The figure shows three views and two pictorial views of one solid part (mm, origin at its lowest corner). Answer the questions. A direction names the side the tool comes from. Coordinates: 2 decimals unless noted, no trailing zeros. Loops run counter-clockwise (first coordinate to the right, second up) from the corner with the lowest first, then second, coordinate; pieces in that order, holes last. Notation, with made-up numbers: M 79,16.25 L 94,16.25 A25 cw 94,51.25 Z; hole C 18,-11 d8. An arc over 180 degrees is marked long. Write each question's results on one line, items separated by ' | '.
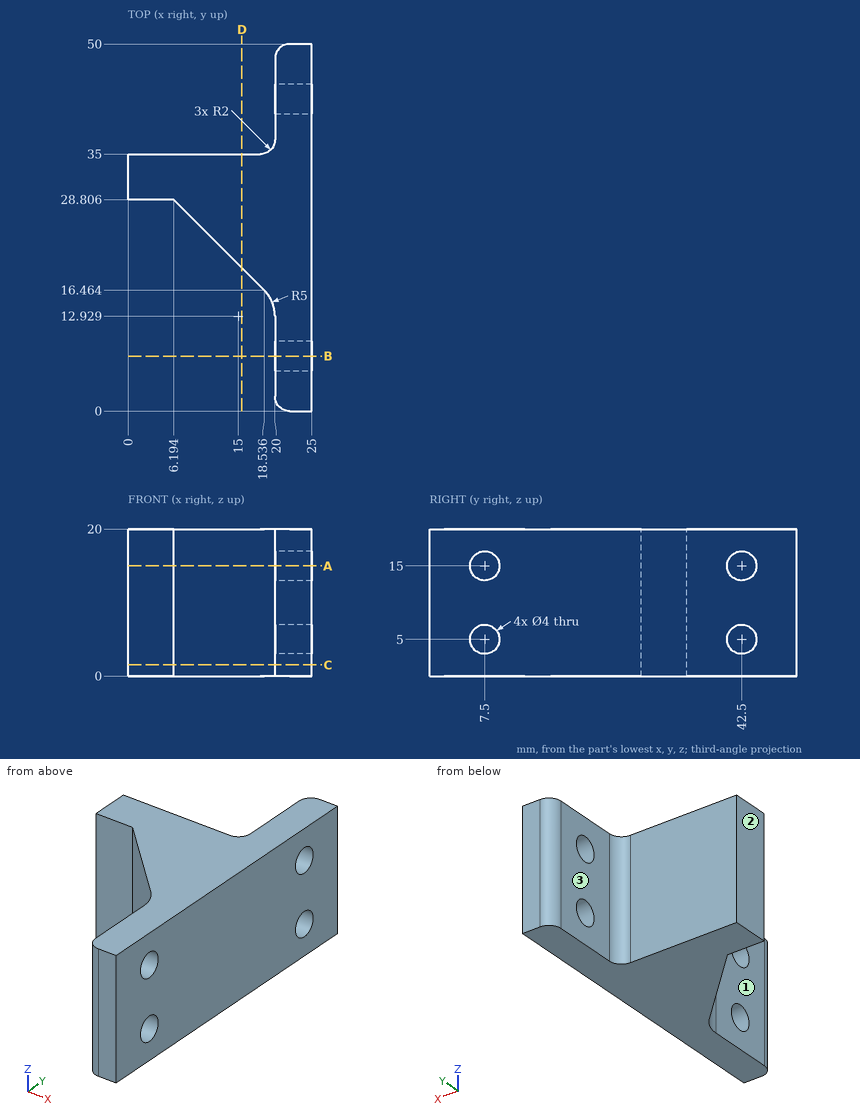
1) Find section B-B, the plane y = 7.5. Give the vertices of the cut face in (x, z).
Check result:
outline: M 20,0 L 25,0 L 25,3 L 20,3 Z; M 20,7 L 25,7 L 25,13 L 20,13 Z; M 20,17 L 25,17 L 25,20 L 20,20 Z
2) Find section D-D, the plane x = 15.5. Give the vertices of the cut face in (y, z).
Check result:
outline: M 19.5,0 L 35,0 L 35,20 L 19.5,20 Z
3) Find section C-C, the plane z = 1.5. Give the vertices of the cut face in (x, y) (1 decimal).
Check result:
outline: M 0,28.8 L 6.2,28.8 L 18.5,16.5 A5 cw 20,12.9 L 20,2 A2 ccw 22,0 L 25,0 L 25,50 L 22,50 A2 ccw 20,48 L 20,37 A2 cw 18,35 L 0,35 Z
4) Given pin 1 Ø12 at (y, z) = (8, 14) entering from -X; pin 2 Ø5 at (x, z) = (3.5, 10) entering from -Y; pin 3 Ø8 at (x, z) = (15, 13.5) entering from -Y, each flat-ended and moving along its own axis, determine where each tip first touches the part or whether it passes through.
Check result:
pin 1: x = 19.88 | pin 2: y = 28.81 | pin 3: y = 15.93
5) Straight lines are drawn through the part: probe 1 along Z at (x, y) = (21.75, 42.5); probe 2 along Y at (x, z) = (3, 5.5) (1 decimal); probe 3 along X at (y, z) = (38.5, 5.5). For each, find the intervals that lie inside material, in ascending order. Write a range as [from, to].
Check result:
probe 1: [0, 3], [7, 13], [17, 20] | probe 2: [28.8, 35] | probe 3: [20, 25]
6) Which of the six approach directions +Z, -Z, +X, -X, +Y, -Y give full straight-line access (tool end or side, diameter ignored) to the marked faces 1, 2 and 3?
Check result:
face 1: +Z, -Z, -X, -Y | face 2: +Z, -Z, -X, +Y, -Y | face 3: +Z, -Z, -X, +Y
7) Find section A-A, the plane z = 15. Give the vertices of the cut face in (x, y) (1 decimal), and give its area (3 significant figures).
Check result:
outline: M 0,28.8 L 6.2,28.8 L 18.5,16.5 A5 cw 20,12.9 L 20,9.5 L 25,9.5 L 25,40.5 L 20,40.5 L 20,37 A2 cw 18,35 L 0,35 Z; M 20,2 A2 ccw 22,0 L 25,0 L 25,5.5 L 20,5.5 Z; M 20,44.5 L 25,44.5 L 25,50 L 22,50 A2 ccw 20,48 Z | area: 429 mm^2
